from build123d import *

# Parameters (mm, degrees)
SKETCH_1_W          = 10
SKETCH_1_H          = 10
SKETCH_1_W_2        = 8
SKETCH_1_H_2        = 8
EXTRUDE_1_DEPTH     = 133.5
SKETCH_2_R          = 1.5
CUT_EXTRUDE_1_DEPTH = 20
SKETCH_3_R          = 1.5
CUT_EXTRUDE_2_DEPTH = 40


with BuildPart() as part:
    # 草图1 → 凸台-拉伸1 (new, symmetric)
    with BuildSketch(Plane.XY):
        Rectangle(SKETCH_1_W, SKETCH_1_H)
        Rectangle(SKETCH_1_W_2, SKETCH_1_H_2, mode=Mode.SUBTRACT)
    extrude(amount=EXTRUDE_1_DEPTH, both=True)

    # 草图2 → 切除-拉伸1 (cut, symmetric)
    with BuildSketch(Plane.XZ.offset(5)):
        with Locations((0, 118.5)):
            Circle(SKETCH_2_R)
        with Locations((0, 98.5)):
            Circle(SKETCH_2_R)
        with Locations((0, 78.5)):
            Circle(SKETCH_2_R)
    extrude(amount=CUT_EXTRUDE_1_DEPTH, both=True, mode=Mode.SUBTRACT)

    # 草图3 → 切除-拉伸2 (cut)
    with BuildSketch(Plane.ZY.offset(5)):
        with Locations(Location((-60, 0, 0), (0, 0, 270))):
            Circle(SKETCH_3_R)
        with Locations(Location((5, 0, 0), (0, 0, 270))):
            Circle(SKETCH_3_R)
    extrude(amount=-CUT_EXTRUDE_2_DEPTH, mode=Mode.SUBTRACT)


solid = part.part
The listing builds one solid part. Answer for the finished solid, in the listing's coordinates (mm). A direction names the side the tool comes from. Round coordinates to 2 decimals unless told otherwise and drop trailing zeros. Order: outer loops, then holes, each group sorted by start corner. A loop starts at its lowest first (then second) coordinate and runs counter-clockwise, first axis right, second up. Notation, with made-up numbers: (89.25, 79.5) -> (136.25, 79.5) arc R18 ccw to (136.25, 109.5) -> close; hole circle Ø4 at (60.25, 16.5). An arc over 180 degrees is marked (long way). Write each question's results on one line, items separated by ' | '. Start each with the question number.
Q1. The mould has two halves that part along X. Classify faces 1 (the flat face through (-4.5, 0.1, 133.5)), 2 (the flat face through (0, -4, 2)), 3 (the flat face through (4, 0, 2)), 4 (the flat face through (5, 0, 2)): pulls with the +X half, pulls with the -X half, needs draft (parallel to the pull), parting line crosses it, or undercut.
Q2. Find section B-B (x = 0). Give the number of separate pieces and of enclosed holes in the cut face, then the cut area to 3 significant figures.
Q3. Find section A-A (y = 0). Determine the outline of the cut face in (x, z), then the cut area to 3 significant figures.
Q4. Find section C-C (z = -109.5). Determine the outline of the cut face in (x, y), then the cut area to 3 significant figures.
Q5. Which of the six approach directions +Z, -Z, +X, -X, +Y, -Y give full straight-line access (tool end or side, diameter ignored) to faces 5 (the flat face through (-4, 0, 2)), 6 (the flat face through (-4.5, 0.1, -133.5))?
Q6. Straight lines are drawn through the part: probe 1 along Z at (x, y) = (0, 4.2); probe 2 along Z at (x, y) = (-4.65, 0); probe 3 along Y at (x, z) = (0.25, 107). For each, find the intervals that lie inside material, in ascending order. Write a range as from..to.
Worked answers:
1) face 1: needs draft | face 2: undercut | face 3: undercut | face 4: pulls with the +X half
2) separate pieces: 8 | enclosed holes: 0 | area: 516 mm2
3) outline: (-5, -133.5) -> (-4, -133.5) -> (-4, -61.5) -> (-5, -61.5) -> close; (-5, -58.5) -> (-4, -58.5) -> (-4, 3.5) -> (-5, 3.5) -> close; (-5, 6.5) -> (-4, 6.5) -> (-4, 133.5) -> (-5, 133.5) -> close; (4, -133.5) -> (5, -133.5) -> (5, -61.5) -> (4, -61.5) -> close; (4, -58.5) -> (5, -58.5) -> (5, 3.5) -> (4, 3.5) -> close; (4, 6.5) -> (5, 6.5) -> (5, 133.5) -> (4, 133.5) -> close | area: 522 mm2
4) outline: (-5, -5) -> (5, -5) -> (5, 5) -> (-5, 5) -> close; hole (-4, -4) -> (4, -4) -> (4, 4) -> (-4, 4) -> close | area: 36.0 mm2
5) face 5: +Z, -Z | face 6: -Z, +X, -X, +Y, -Y
6) probe 1: z = -133.5..77, 80..97, 100..117, 120..133.5 | probe 2: z = -133.5..-61.5, -58.5..3.5, 6.5..133.5 | probe 3: y = -5..-4, 4..5
